from build123d import *

# Parameters (mm, degrees)
SKETCH2_W           = 25.4
SKETCH2_H           = 50.8
BOSS_EXTRUDE1_DEPTH = 2.00000108
SKETCH3_W           = 23.39999892
SKETCH3_H           = 48.79999892
SKETCH3_W_2         = 21.39999784
SKETCH3_H_2         = 46.79999784
BOSS_EXTRUDE2_DEPTH = 4.999999906
FILLET1_R           = 2.000000064
FILLET2_R           = 1.000000032
CUT_EXTRUDE2_REACH  = 51.8
SKETCH5_R           = 2.2225
CUT_EXTRUDE3_REACH  = 51.8
SKETCH6_W           = 7.62
SKETCH6_H           = 3.81
CUT_EXTRUDE4_REACH  = 26.4
SKETCH7_W           = 2.54
SKETCH7_H           = 2.54


with BuildPart() as part:
    # Sketch2 → Boss-Extrude1 (new body)
    with BuildSketch(Plane.XY):
        with Locations((12.7, 25.4)):
            Rectangle(SKETCH2_W, SKETCH2_H)
    extrude(amount=BOSS_EXTRUDE1_DEPTH)

    # Sketch3 → Boss-Extrude2 (add)
    with BuildSketch(Plane.XY.offset(2.00000108)):
        with Locations((12.7, 25.4)):
            Rectangle(SKETCH3_W, SKETCH3_H)
        with Locations((12.7, 25.4)):
            Rectangle(SKETCH3_W_2, SKETCH3_H_2, mode=Mode.SUBTRACT)
    extrude(amount=BOSS_EXTRUDE2_DEPTH)

    # Fillet1
    fillet1_edges = [part.edges().sort_by_distance(p)[0] for p in [
        (0, 50.8, 1.00000054),
        (25.4, 50.8, 1.00000054),
        (25.4, 0, 1.00000054),
        (0, 0, 1.00000054),
    ]]
    fillet(fillet1_edges, radius=FILLET1_R)

    # Fillet2
    fillet2_edges = [part.edges().sort_by_distance(p)[0] for p in [
        (0, 25.4, 0),
        (12.7, 50.8, 0),
        (25.4, 25.4, 0),
        (12.7, 0, 0),
        (24.814213544, 50.214213544, 0),
        (24.814213544, 0.585786456, 0),
        (0.585786456, 0.585786456, 0),
        (0.585786456, 50.214213544, 0),
    ]]
    fillet(fillet2_edges, radius=FILLET2_R)

    # Sketch5 → Cut-Extrude2 (cut, up to next)
    with BuildSketch(Plane.XZ.offset(-1.00000054), mode=Mode.PRIVATE) as cut_extrude2_sk1:
        with Locations((18.319999936, 4.54000108)):
            Circle(SKETCH5_R)
    cut_extrude2_tool1 = extrude(cut_extrude2_sk1.sketch, amount=-CUT_EXTRUDE2_REACH, mode=Mode.PRIVATE) & part.part
    add(cut_extrude2_tool1.solids().sort_by_distance((18.32, 1.000001, 4.540001))[0], mode=Mode.SUBTRACT)

    # Sketch6 → Cut-Extrude3 (cut, up to next)
    with BuildSketch(Plane.XZ.offset(-1.00000054), mode=Mode.PRIVATE) as cut_extrude3_sk1:
        with Locations((10.699999936, 3.90500108)):
            Rectangle(SKETCH6_W, SKETCH6_H)
    cut_extrude3_tool1 = extrude(cut_extrude3_sk1.sketch, amount=-CUT_EXTRUDE3_REACH, mode=Mode.PRIVATE) & part.part
    add(cut_extrude3_tool1.solids().sort_by_distance((10.7, 1.000001, 3.905001))[0], mode=Mode.SUBTRACT)

    # Sketch7 → Cut-Extrude4 (cut, up to next)
    with BuildSketch(Plane.ZY.offset(-1.00000054), mode=Mode.PRIVATE) as cut_extrude4_sk1:
        with Locations((3.27000108, 10.890000064)):
            Rectangle(SKETCH7_W, SKETCH7_H)
    cut_extrude4_tool1 = extrude(cut_extrude4_sk1.sketch, amount=-CUT_EXTRUDE4_REACH, mode=Mode.PRIVATE) & part.part
    add(cut_extrude4_tool1.solids().sort_by_distance((1.000001, 10.89, 3.270001))[0], mode=Mode.SUBTRACT)
    # Sketch7 → Cut-Extrude4 (cut, up to next)
    with BuildSketch(Plane.ZY.offset(-1.00000054), mode=Mode.PRIVATE) as cut_extrude4_sk2:
        with Locations((3.27000108, 21.050000064)):
            Rectangle(SKETCH7_W, SKETCH7_H)
    cut_extrude4_tool2 = extrude(cut_extrude4_sk2.sketch, amount=-CUT_EXTRUDE4_REACH, mode=Mode.PRIVATE) & part.part
    add(cut_extrude4_tool2.solids().sort_by_distance((1.000001, 21.05, 3.270001))[0], mode=Mode.SUBTRACT)


solid = part.part
Design review of the part built by this model. Coordinates are the model's own, in mm. A direction names the side the tool comes from. Round coordinates to 2 decimals unless told otherwise and drop trailing zeros. Write each loop counter-clockwise with the first axis right and the second up, starting at its lowest first coordinate (ties: lowest second). Pieces come first, ordered by that corner, then holes. Notation, with made-up numbers: (35.5, -5.5) -> (56.5, -5.5) arc R26 cw to (56.5, 21.5) -> close; hole circle Ø5 at (77, 23.25). An arc over 180 degrees is marked (long way). One line per item, written item: value. Start each with the question number.
Q1. Add section A-A (x = 18.32). Give the boundary of the cut face in (y, z), then the cut area to 3 significant figures.
Q2. Tool access review of faces 1 (the face through (1.5, 10.9, 4.54)), 2 (the face through (23.4, 25, 4)), 3 (the face through (24.4, 25, 4)): name each direction out of +Z, -Z, +X, -X, +Y, -Y from which nothing blocks a thin tool from reaching the whole face with its end or side.
Q3. The part is to be moulded in two halves that separate along X. For faces 4 (the face through (0.57, 50.2, 1.51)), 5 (the face through (13, 49.8, 4)), 6 (the face through (2, 25, 4)), say which applies: pulls with the +X half, pulls with the -X half, needs draft (parallel to the pull), parting line crosses it, or undercut.
Q4. Insertion check: P1, Ø0.5, axis at x = 12.5, y = 1.5, coming from the -Z side; P2, Ø1.5, axis at y = 21.5, z = 4, coming from the +X side; P3, Ø1.1, axis at x = 1.5, z = 4, coming from the +Y side; P4, Ø2.5, axis at x = 8, z = 4, coming from the -Y side. Each pin has a flat end and moves straight along its axis. Give the tip position at first contact, or say it passes through.
Q5. Add section C-C (x = 5.5). Give the boundary of the cut face in (y, z).
Q6. Add section B-B (y = 18). Give the boundary of the cut face in (x, z).
Q7. Add section D-D (x = 8.5). Give the boundary of the cut face in (y, z), then the cut area to 3 significant figures.
Q8. To check wall thickness, follow probe 1 along X at (y, z) = (16.5, 4.5); probe 2 along Z at (x, y) = (18.32, 1.8); probe 3 along Y at (x, z) = (20.75, 2.75). State the ranges of each line that lie inside material, in increasing order.
Response:
1. outline: (0, 1) arc R1 ccw to (1, 0) -> (49.8, 0) arc R1 ccw to (50.8, 1) -> (50.8, 2) -> (49.8, 2) -> (49.8, 7) -> (48.8, 7) -> (48.8, 2) -> (2, 2) -> (2, 2.32) -> (1, 2.32) -> (1, 2) -> (0, 2) -> close; (1, 6.76) -> (2, 6.76) -> (2, 7) -> (1, 7) -> close
1. area: 107 mm^2
2. face 1: -X
2. face 2: +Z
2. face 3: +Z, +X, +Y, -Y
3. face 4: pulls with the -X half
3. face 5: needs draft
3. face 6: undercut
4. P1: stops at z = 0
4. P2: stops at x = 24.4
4. P3: stops at y = 49.8
4. P4: stops at y = 1
5. outline: (0, 1) arc R1 ccw to (1, 0) -> (49.8, 0) arc R1 ccw to (50.8, 1) -> (50.8, 2) -> (49.8, 2) -> (49.8, 7) -> (48.8, 7) -> (48.8, 2) -> (2, 2) -> (2, 7) -> (1, 7) -> (1, 2) -> (0, 2) -> close
6. outline: (0, 1) arc R1 ccw to (1, 0) -> (24.4, 0) arc R1 ccw to (25.4, 1) -> (25.4, 2) -> (24.4, 2) -> (24.4, 7) -> (23.4, 7) -> (23.4, 2) -> (2, 2) -> (2, 7) -> (1, 7) -> (1, 2) -> (0, 2) -> close
7. outline: (0, 1) arc R1 ccw to (1, 0) -> (49.8, 0) arc R1 ccw to (50.8, 1) -> (50.8, 2) -> (49.8, 2) -> (49.8, 7) -> (48.8, 7) -> (48.8, 2) -> (0, 2) -> close; (1, 5.81) -> (2, 5.81) -> (2, 7) -> (1, 7) -> close
7. area: 107 mm^2
8. probe 1: x = 1 to 2, 23.4 to 24.4
8. probe 2: z = 0 to 2.32, 6.76 to 7
8. probe 3: y = 1 to 2, 48.8 to 49.8
